Autodesk Inventor part; units mm, degrees
ref_plane "YZ Plane" through (0, 0, 0) normal (1, 0, 0) x (0, 1, 0)
ref_plane "XZ Plane" through (0, 0, 0) normal (0, 1, 0) x (-1, 0, 0)
ref_plane "XY Plane" through (0, 0, 0) normal (0, 0, 1) x (1, 0, 0)
sketch "Sketch1" plane through (0, 0, 0) normal (0, 1, 0) x (-1, 0, 0)
  circle A0 centre (0, 0) radius 17.5
  arc A1 (13.975, 14.3073) -> (13.975, -14.3073) centre (0, 0) ccw
  line L0 (13.975, 14.3073) -> (13.975, 17.5)
  line L1 (13.975, 17.5) -> (19.5, 17.5)
  line L2 (19.5, 17.5) -> (19.5, 0)
  line L3 (0, 0) -> (32.178, 0) construction
  line L4 (13.975, -14.3073) -> (13.975, -17.5)
  line L5 (13.975, -17.5) -> (19.5, -17.5)
  line L6 (19.5, -17.5) -> (19.5, 0)
  dimension "d0" = 35
  dimension "d2" = 19.5
  dimension "d3" = 17.5
  dimension "d4" = 5.525
  dimension "d5" = 13.975
  dimension "d6" = 40
extrude "Extrusion1" add sketch "Sketch1" along normal mid plane 20
sketch "Sketch2" plane through (-19.5, -10, 17.5) normal (-1, 0, 0) x (0, 0, 1)
  circle A0 centre (-33, 10) radius 1.25
  circle A1 centre (-2, 10) radius 1.25
  line L0 (0, 0) -> (-35, 0)
  point P0 (-17.5, 10)
  dimension "d14" = 31
  dimension "d15" = 15.5
  dimension "d16" = 2.5
  dimension "d17" = 2.5
  dimension "d18" = 10
  dimension "d19" = 10
extrude "Extrusion2" add sketch "Sketch2" along normal blind 10
properties part number "motor-hold"
Can you work these out from the model? Positions are in its coordinate system, mm. A direction names the side the tool comes from. Give positions to 0.01 mm unless a question says otherwise; leave off trailing zeros. Write each loop counter-clockwise with the first axis right and the second up, starting at its lowest first coordinate (ties: lowest second). Pieces come first, ordered by that corner, then holes. Notation, with made-up numbers: (33.25, 75.5) -> (39.25, 75.5) arc R24 ccw to (39.25, 114.5) -> close; hole circle Ø11 at (39.25, -15.75). An arc over 180 degrees is marked (long way). Answer as a JSON object with one key per item and string values. Group by question number.
Item 1: We'd pull the mould along X, two halves only. Please class faces 1 (the face through (-13.975, 0, 16)), 2 (the face through (-29.5, 0, -16)), 3 (the face through (-24.43, -0.05, -16.75)): +X half, -X half, draft (parallel to the pull), parting line (faces both ways), or undercut.
Item 2: Suppose I cut it at C-C (z = 15.5). Please give me the cut outline in (x, y) (3 decimals), plus the area to 3 significant figures.
Item 3: For faces 4 (the face through (-24.43, -0.05, 14.25)), 5 (the face through (-17, 0, -17.5)), 6 (the face through (-17, 0, 17.5)), which set-ups out of +Z, -Z, +X, -X, +Y, -Y let a thin tool reach every point of the face, with its end or its side?
Item 4: Suppose I cut it at B-B (y = 7.75). Please give me the cut outline in (x, z) (3 decimals), plus the area to 3 significant figures.
Item 5: I'm going to push flat-ended pins straight in: P1, Ø12, axis at y = 4.5, z = -8.5, coming from the -X side; P2, Ø3, axis at x = -16.5, y = 2, coming from the +Z side; P3, Ø5, axis at x = 7.5, y = -7.5, coming from the -Z side. Where does each tip first touch, or does it pass through?
Item 6: Suppose I cut it at D-D (x = -3). Please give me the cut outline in (y, z).
Item 7: Suppose I cut it at A-A (z = 0). Please give me the cut outline in (x, y).
Item 8: Please list where these lines run through material, in increasing order: line 1 (Z direction, x = 0, y = -2.75); line 2 (X direction, y = -2, z = 16) (3 decimals); line 3 (X direction, y = 4.75, z = 4). Write a range as [from, to].
Findings:
{
 "1": {"face 1": "undercut", "face 2": "-X half", "face 3": "draft"},
 "2": {"outline": "(-29.5, -1.25) -> (-19.5, -1.25) -> (-19.5, -10) -> (-13.975, -10) -> (-13.975, 10) -> (-19.5, 10) -> (-19.5, 1.25) -> (-29.5, 1.25) -> close; (-12.639, -10) -> (-8.124, -10) -> (-8.124, 10) -> (-12.639, 10) -> close; (8.124, -10) -> (12.639, -10) -> (12.639, 10) -> (8.124, 10) -> close", "area": "316 mm²"},
 "3": {"face 4": "-X", "face 5": "-Z, -X, +Y, -Y", "face 6": "+Z, -X, +Y, -Y"},
 "4": {"outline": "(-19.5, -17.5) -> (-13.975, -17.5) -> (-13.975, -14.307) arc R20 ccw (long way) to (-13.975, 14.307) -> (-13.975, 17.5) -> (-19.5, 17.5) -> close; hole circle Ø35 at (0, 0)", "area": "369 mm²"},
 "5": {"P1": "stops at x = -19.5", "P2": "stops at z = 17.5", "P3": "stops at z = -19.36"},
 "6": {"outline": "(-10, -19.77) -> (10, -19.77) -> (10, -17.24) -> (-10, -17.24) -> close; (-10, 17.24) -> (10, 17.24) -> (10, 19.77) -> (-10, 19.77) -> close"},
 "7": {"outline": "(-19.5, -10) -> (-17.5, -10) -> (-17.5, 10) -> (-19.5, 10) -> close; (17.5, -10) -> (20, -10) -> (20, 10) -> (17.5, 10) -> close"},
 "8": {"line 1": "z = [-20, -17.5], [17.5, 20]", "line 2": "x = [-19.5, -13.975], [-12, -7.089], [7.089, 12]", "line 3": "x = [-19.5, -17.04], [17.04, 19.6]"}
}
